Here's the drawing with two shaded views (mm, measured from the low corner). I have some questions. Coordinates: 2 decimals unless noted, no trailing zeros. Loops run counter-clockwise (first coordinate to the right, second up) from the corner with the lowest first, then second, coordinate; pieces in that order, holes last. Notation, with made-up numbers: M 51.5,32.25 L 106.5,32.25 A19 ccw 106.5,55.25 Z; hole C 31,60.25 d4. An arc over 180 degrees is marked long. Return JSON: item names as keys, results as strings. Group by question number.
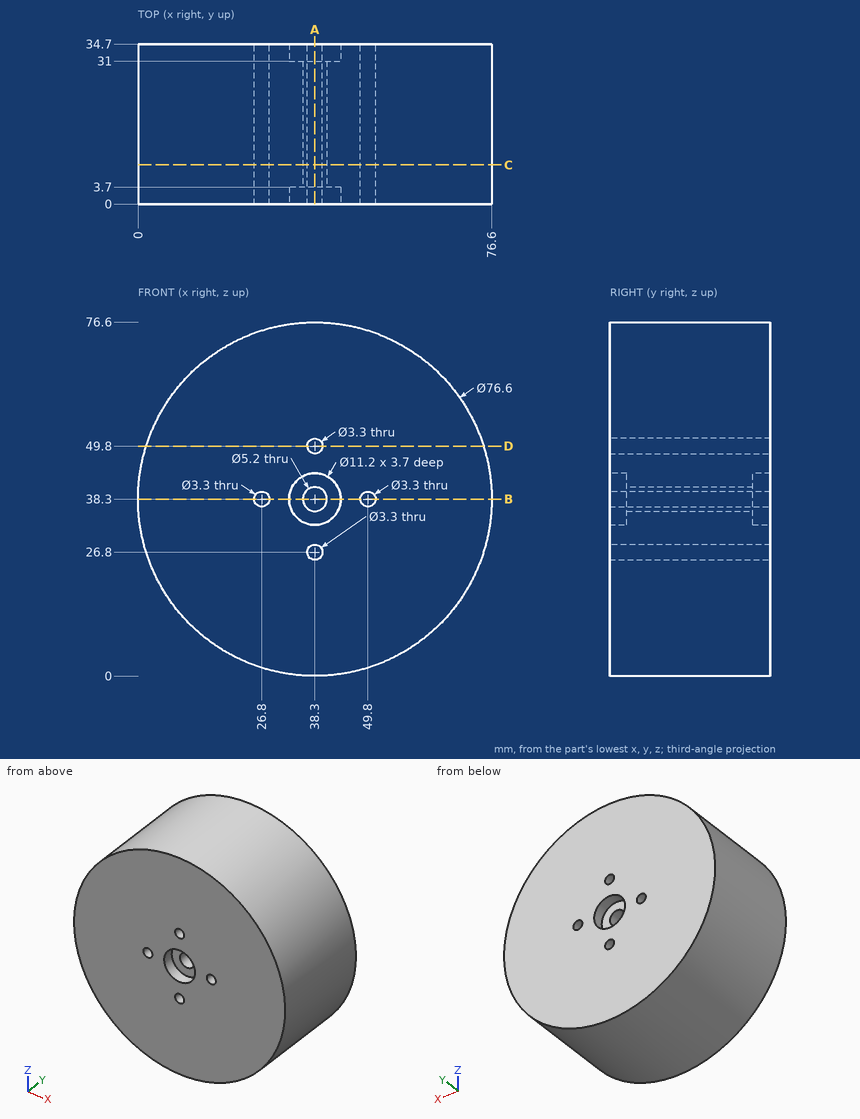
(1) Will these pins go through, and if not, where does the flat tip stop? P1, Ø4, axis at x = 33, y = 27, coming from the +Z side; P2, Ø12, axis at x = 51, y = 26, coming from the -Z side; P3, Ø3.5, axis at x = 36, z = 38, coming from the +Y side; P4, Ø3, axis at x = 38.3, z = 38.3, coming from the -Y side.
(2) Imagine slicing it at C-C, the plane y = 8.5. Write out the boundary of the cut face in (x, z).
(3) Imagine slicing it at A-A, the plane x = 38.3. Write out the boundary of the cut face in (y, z), then the cut area to 3 significant figures.
(4) If I drill on L1, parallel to Z at x = 38, y = 25; L2, parallel to Z at x = 50.5, y = 27; L3, parallel to Z at x = 36, y = 3.5, over which ranges is the centre line in solid material (lowest first)? Write a range as [from, to].
(5) Imagine slicing it at B-B, the plane z = 38.3. Write out the boundary of the cut face in (x, y), then the cut area to 3 significant figures.
(6) Imagine slicing it at D-D, the plane z = 49.8. Write out the boundary of the cut face in (x, y).
Checks:
{
 "1": {"P1": "z = 76.46", "P2": "z = 0.59", "P3": "y = 31", "P4": "through"},
 "2": {"outline": "C 38.3,38.3 d76.6; hole C 26.8,38.3 d3.3; hole C 38.3,38.3 d5.2; hole C 38.3,26.8 d3.3; hole C 38.3,49.8 d3.3; hole C 49.8,38.3 d3.3"},
 "3": {"outline": "M 0,0 L 34.7,0 L 34.7,25.15 L 0,25.15 Z; M 0,28.45 L 34.7,28.45 L 34.7,32.7 L 31,32.7 L 31,35.7 L 3.7,35.7 L 3.7,32.7 L 0,32.7 Z; M 0,43.9 L 3.7,43.9 L 3.7,40.9 L 31,40.9 L 31,43.9 L 34.7,43.9 L 34.7,48.15 L 0,48.15 Z; M 0,51.45 L 34.7,51.45 L 34.7,76.6 L 0,76.6 Z", "area": "2,200 mm²"},
 "4": {"L1": "[0, 25.18], [28.42, 35.72], [40.88, 48.18], [51.42, 76.6]", "L2": "[2, 36.81], [39.79, 74.6]", "L3": "[0.07, 33.19], [43.41, 76.53]"},
 "5": {"outline": "M 0,0 L 25.15,0 L 25.15,34.7 L 0,34.7 Z; M 28.45,0 L 32.7,0 L 32.7,3.7 L 35.7,3.7 L 35.7,31 L 32.7,31 L 32.7,34.7 L 28.45,34.7 Z; M 40.9,3.7 L 43.9,3.7 L 43.9,0 L 48.15,0 L 48.15,34.7 L 43.9,34.7 L 43.9,31 L 40.9,31 Z; M 51.45,0 L 76.6,0 L 76.6,34.7 L 51.45,34.7 Z", "area": "2,200 mm²"},
 "6": {"outline": "M 1.77,0 L 36.65,0 L 36.65,34.7 L 1.77,34.7 Z; M 39.95,0 L 74.83,0 L 74.83,34.7 L 39.95,34.7 Z"}
}
